```python
from build123d import *

# Parameters (mm, degrees)
BOSS_EXTRU_1_DEPTH      = 5
ESQUISSE2_W             = 20
ESQUISSE2_H             = 20
ENL_V_MAT_EXTRU_1_DEPTH = 5
ENL_V_MAT_EXTRU_2_DEPTH = 5
CONG_1_R                = 3


with BuildPart() as part:
    # Esquisse1 → Boss.-Extru.1 (new body)
    with BuildSketch(Plane.XY):
        Polygon((-112.248737342, -130), (-87.5, -154.748737342), (87.5, -154.748737342), (112.248737342, -130), (112.248737342, 130), (87.5, 154.748737342), (-87.5, 154.748737342), (-112.248737342, 130), align=None)
    extrude(amount=BOSS_EXTRU_1_DEPTH)

    # Esquisse2 → Enlèv. mat.-Extru.1 (cut)
    with BuildSketch(Plane.XY.offset(5)):
        with Locations((-65, 131.748737342)):
            Rectangle(ESQUISSE2_W, ESQUISSE2_H)
        with Locations((-65, -131.748737342)):
            Rectangle(ESQUISSE2_W, ESQUISSE2_H)
        with Locations((65, -131.748737342)):
            Rectangle(ESQUISSE2_W, ESQUISSE2_H)
        with Locations((65, 131.748737342)):
            Rectangle(ESQUISSE2_W, ESQUISSE2_H)
    extrude(amount=-ENL_V_MAT_EXTRU_1_DEPTH, mode=Mode.SUBTRACT)

    # Esquisse3 → Enlèv. mat.-Extru.2 (cut)
    with BuildSketch(Plane.XY.offset(5)):
        Polygon((-87.5, 154.748737342), (-112.248737342, 130), (-112.248737342, -130), (-87.5, -154.748737342), (87.5, -154.748737342), (112.248737342, -130), (112.248737342, 130), (87.5, 154.748737342), align=None)
        Polygon((-107.248737342, 127.928932188), (-107.248737342, -127.928932188), (-85.428932188, -149.748737342), (85.428932188, -149.748737342), (107.248737342, -127.928932188), (107.248737342, 127.928932188), (85.428932188, 149.748737342), (-85.428932188, 149.748737342), align=None, mode=Mode.SUBTRACT)
    extrude(amount=-ENL_V_MAT_EXTRU_2_DEPTH, mode=Mode.SUBTRACT)

    # Congé1
    cong_1_edges = [part.edges().sort_by_distance(p)[0] for p in [
        (-85.428932188, 149.748737342, 2.5),
        (85.428932188, 149.748737342, 2.5),
        (107.248737342, 127.928932188, 2.5),
        (107.248737342, -127.928932188, 2.5),
        (85.428932188, -149.748737342, 2.5),
        (-85.428932188, -149.748737342, 2.5),
        (-107.248737342, -127.928932188, 2.5),
        (-107.248737342, 127.928932188, 2.5),
    ]]
    fillet(cong_1_edges, radius=CONG_1_R)


solid = part.part
```
Can you work these out from the model? Positions are in its coordinate system, mm. Give positions to 0.01 mm unless a question says otherwise; leave off trailing zeros. Loops run counter-clockwise (first coordinate to the right, second up) from the corner with the lowest first, then second, coordinate; pieces in that order, holes last. Notation, with made-up numbers: M 73.5,34 L 88.5,34 A25 cw 88.5,59 Z; hole C 0,57.5 d5. An arc over 180 degrees is marked long. Answer in a Markdown table with one row per item.
1. If I drill on line 1 along Y through (x, z) = (-66, 2.6); line 2 along Y through (x, z) = (-92, 3.15); line 3 along Y through (x, z) = (-86, 2.7), over which ranges is the centre line in solid material (lowest first)?
Taken from the geometry:
| item | result |
|---|---|
| line 1 | y = -149.75 to -141.75, -121.75 to 121.75, 141.75 to 149.75 |
| line 2 | y = -143.18 to 143.18 |
| line 3 | y = -149.14 to 149.14 |
2. Suppose I cut it at A-A on x = -68. Write out the boundary of the cut face in (y, z).
Taken from the geometry:
| item | result |
|---|---|
| outline | M -149.75,0 L -141.75,0 L -141.75,5 L -149.75,5 Z; M -121.75,0 L 121.75,0 L 121.75,5 L -121.75,5 Z; M 141.75,0 L 149.75,0 L 149.75,5 L 141.75,5 Z |
3. For pin 1 Ø1.5 at (y, z) = (134, 2) entering from -X; pin 2 Ø1.5 at (y, z) = (-131, 1.5) entering from +X; pin 3 Ø2.5 at (y, z) = (135.5, 3.5) entering from -X, each with a flat end and sliding along its axis, tell me the tip position at first contact or that it passes through.
Taken from the geometry:
| item | result |
|---|---|
| pin 1 | stops at x = -101.93 |
| pin 2 | stops at x = 104.93 |
| pin 3 | stops at x = -100.93 |
4. Suppose I cut it at B-B on z = 1.1. Count the separate pieces of the cut face and the enclosed holes in it, plus the area to 3 significant figures.
Taken from the geometry:
| item | result |
|---|---|
| separate pieces | 1 |
| enclosed holes | 4 |
| area | 61,700 mm² |
5. Suppose I cut it at C-C on x = 91. Write out the boundary of the cut face in (y, z).
Taken from the geometry:
| item | result |
|---|---|
| outline | M -144.18,0 L 144.18,0 L 144.18,5 L -144.18,5 Z |
